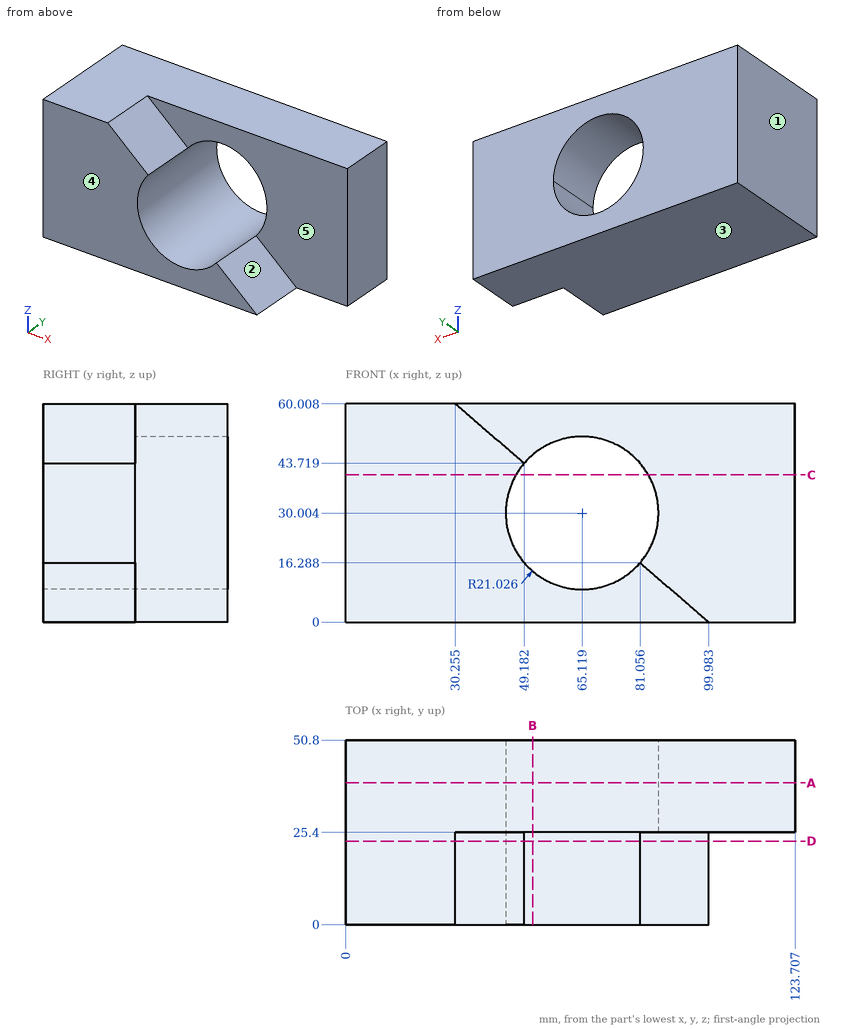
Here's the drawing with two shaded views (mm, measured from the low corner). I have some questions. A direction names the side the tool comes from. Give positions to 0.01 mm unless a question says otherwise; leave off trailing zeros. Loops run counter-clockwise (first coordinate to the right, second up) from the corner with the lowest first, then second, coordinate; pieces in that order, holes last. Notation, with made-up numbers: (-24.75, -29.5) -> (-0.75, -29.5) arc R32 cw to (-0.75, 4.5) -> close; hole circle Ø1 at (-27, 77). An arc over 180 degrees is marked (long way). Use one line per item in the form item = value.
1) For the marked faces 4 and 5, which set-ups out of +Z, -Z, +X, -X, +Y, -Y let a thin tool reach every point of the face, with its end or its side?
Answers:
face_4 = +Z, -Z, +X, -X, -Y
face_5 = +Z, +X, -Y
2) If we section it at C-C (z = 40.5): Please give me the cut outline in (x, y), plus the area to 3 significant figures.
Answers:
outline = (0, 0) -> (46.9, 0) -> (46.9, 50.8) -> (0, 50.8) -> close; (83.34, 25.4) -> (123.71, 25.4) -> (123.71, 50.8) -> (83.34, 50.8) -> close
area = 3,410 mm²
3) If we section it at B-B (x = 51.5): Please give me the cut outline in (y, z) (1 decimal).
Answers:
outline = (0, 0) -> (50.8, 0) -> (50.8, 14) -> (0, 14) -> close; (25.4, 46) -> (50.8, 46) -> (50.8, 60) -> (25.4, 60) -> close
4) If we section it at D-D (y = 23): Please give me the cut outline in (x, z) (1 decimal), plus the area to 3 significant figures.
Answers:
outline = (0, 0) -> (100, 0) -> (81.1, 16.3) arc R21 cw to (49.2, 43.7) -> (30.3, 60) -> (0, 60) -> close
area = 3,210 mm²
5) I need wall thicknesses on line 1 along Y through (x, z) = (51, 51.5); line 2 along Z through (x, y) = (64.5, 27); line 3 along Z through (x, y) = (81, 44.5) (1 decimal). Which ranges of each line are inside material? Lowest first, please.
Answers:
line_1 = 25.4 to 50.8
line_2 = 0 to 8.99, 51.02 to 60.01
line_3 = 0 to 16.2, 43.8 to 60
6) If we section it at A-A (y = 39): Please give me the cut outline in (x, z) (1 decimal), plus the area to 3 significant figures.
Answers:
outline = (0, 0) -> (123.7, 0) -> (123.7, 60) -> (0, 60) -> close; hole circle Ø42.1 at (65.1, 30)
area = 6,030 mm²
7) We'd pull the mould along X, two halves only. Please class the marked faces 1, 2 and 3: released by +X, released by -X, zero draft, split by the parting line, or undercut.
Answers:
face_1 = released by -X
face_2 = released by +X
face_3 = zero draft
8) Will these pins go through, and if not, where does the flat tip stop? pin 1 (6 mm diameter, centred on y = 25.5, z = 44, fed in from -X); pin 2 (1 mm diameter, centred on x = 65.5, z = 54, fed in from -Y).
Answers:
pin_1 = 0
pin_2 = 25.4
